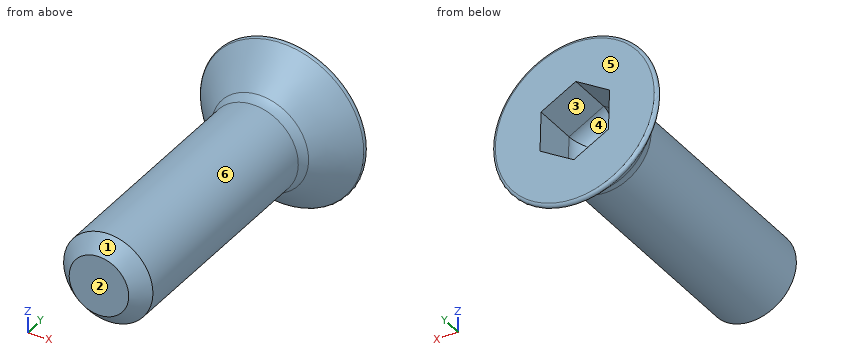
Autodesk Inventor part; units mm, degrees
ref_plane "YZ Plane" through (0, 0, 0) normal (1, 0, 0) x (0, 1, 0)
ref_plane "XZ Plane" through (0, 0, 0) normal (0, 1, 0) x (-1, 0, 0)
ref_plane "XY Plane" through (0, 0, 0) normal (0, 0, 1) x (1, 0, 0)
sketch "Szkic2" plane through (0, 0, 0) normal (1, 0, 0) x (0, 1, 0)
  line L0 (0, -2.9) -> (0, 2.9)
  line L1 (-1.5, -1.5) -> (-1.5, 1.5)
  line L2 (-1.5, -1.5) -> (0, -2.9)
  line L3 (-1.5, 1.5) -> (0, 2.9)
  line L4 (0, 0) -> (-10, 0)
  line L5 (-10, 0) -> (-10, -1.5)
  line L6 (-10, -1.5) -> (-1.5, -1.5)
  dimension "d0" = 5.8
  dimension "d2" = 3
  dimension "d3" = 1.5
  dimension "d4" = 10
  dimension "d5" = 1.5
revolve "Obrót1" add sketch "Szkic2" angle 360 about axis through (0, 0, 0) along (0, -1, 0) contours L2 L1 L4 L0 | L6 L5 L4 L1
sketch "Szkic3" plane through (0, 0, 0) normal (0, 1, 0) x (1, 0, 0)
  line L0 (-1.1673, -0.633) -> (-1.1318, 0.6945)
  line L1 (-1.1318, 0.6945) -> (0.0355, 1.3274)
  line L2 (0.0355, 1.3274) -> (1.1673, 0.633)
  line L3 (1.1673, 0.633) -> (1.1318, -0.6945)
  line L4 (1.1318, -0.6945) -> (-0.0355, -1.3274)
  line L5 (-0.0355, -1.3274) -> (-1.1673, -0.633)
  point P0 (0, 0)
  point P1 (0, 0)
  dimension "d7" = 2.3
extrude "Wyciągnięcie proste1" cut sketch "Szkic3" against normal blind 2
fillet "Zaokrąglenie1" radius 0.5 6 edges at (-1.1496, -2, -0.0308) (-0.6014, -2, 0.9802) (-0.5482, -2, -1.011) (0.6014, -2, -0.9802) (0.5482, -2, 1.011) (1.1496, -2, 0.0308)
fillet "Zaokrąglenie2" radius 0.5 1 edges at (0, -1.5, 1.5)
fillet "Zaokrąglenie3" radius 0.1 1 edges at (0, 0, 2.9)
thread "Gwint1"
chamfer "Faza1" distance 0.5 angle 45 1 edges at (0, -10, 1.5)
properties part number "Screw M3 10mm flat head"
Model file for the job. Use its own axes, mm. Face numbers are marked on the shaded views. A direction names the side the tool comes from. Give positions to 0.01 mm unless a question says otherwise; leave off trailing zeros. Order: outer loops, then holes, each group sorted by start corner. A loop starts at its lowest first (then second) coordinate and runs counter-clockwise, first axis right, second up.
1) Wall check: probe 1 along X at (y, z) = (-2.25, 1.3); probe 2 along X at (y, z) = (-1.5, -1.2); probe 3 along Y at (x, z) = (0.95, 2.1). Give the ranges that are in metal, low to high.
2) Saw through at A-A, the plane y = -8. Write the cut outline in (x, z).
3) Pin check, flat tips, straight feed: pin 1 (2 mm diameter, centred on x = 0, y = -6, fed in from -Z); pin 2 (1.5 mm diameter, centred on y = -5.5, z = 0, fed in from +X); pin 3 (1 mm diameter, centred on x = 0.5, y = -9, fed in from +Z). Stop position of each tip, or through.
4) Mould opens along X. For the marked faces 1, 2, 3 and 4 say: +X half, -X half, draft (parallel to the pull), parting line (faces both ways), or undercut.
5) 3-axis set-ups, long thin cutter, end or side, ignore diameter. For the marked faces 5 and 6: which of +Z, -Z, +X, -X, +Y, -Y reach the whole face in a straight line?
Computed:
1. probe 1: x = -0.75 to 0.75
1. probe 2: x = -0.97 to -0.2, 0.24 to 0.97
1. probe 3: y = -0.64 to 0
2. outline: circle Ø3 at (0, 0)
3. pin 1: stops at z = -1.5
3. pin 2: stops at x = 1.5
3. pin 3: stops at z = 1.5
4. face 1: parting line
4. face 2: draft
4. face 3: undercut
4. face 4: undercut
5. face 5: +Z, -Z, +X, -X, +Y
5. face 6: -Y
